Autodesk Inventor part; units mm, degrees
ref_plane "工作平面2" through (11.9199, 26.93, -12.8525) normal (0, 0, 1) x (-1, 0, 0)
ref_plane "工作平面3" through (0.201, 1.0367, -16.3525) normal (0, 0, -1) x (0, 1, 0)
ref_plane "YZ Plane" through (0, 0, 0) normal (1, 0, 0) x (0, 1, 0)
sketch "草图1" plane through (0, 0, 0) normal (0, 0, 1) x (1, 0, 0)
  line L0 (4.75, -1.5) -> (-4.75, -1.5)
  line L1 (-4.75, -1.5) -> (-4.75, 1.5)
  line L2 (-4.75, 1.5) -> (4.75, 1.5)
  line L3 (4.75, 1.5) -> (4.75, -1.5)
  line L4 (4.75, -1.5) -> (-4.75, 1.5) construction
  line L5 (-4.75, -1.5) -> (4.75, 1.5) construction
  circle A0 centre (0, 0) radius 1
  dimension "d0" = 3
  dimension "d1" = 2
  dimension "d2" = 9.5
extrude "拉伸1" add sketch "草图1" along normal blind 3
sketch "草图2" plane through (0, 0, 3) normal (0, 0, 1) x (1, 0, 0)
  line L0 (4.75, 1.5) -> (-4.75, 1.5)
  line L1 (-4.75, 1.5) -> (-4.75, -1.5)
  line L2 (-4.75, -1.5) -> (4.75, -1.5)
  line L3 (4.75, -1.5) -> (4.75, 1.5)
  circle A0 centre (0, 0) radius 1
extrude "拉伸2" add sketch "草图2" along normal blind 10 contours L3 L2 L1 L0 | A0
sketch "草图3" plane through (-4.75, 1.5, 0) normal (0, 1, 0) x (1, 0, 0)
  line L0 (-1.5, 0) -> (11, 0)
  line L1 (11, 0) -> (11, -7)
  line L2 (11, -7) -> (-1.5, -7)
  line L3 (-1.5, -7) -> (-1.5, 0)
  line L4 (9.5, 0) -> (9.5, -13)
  line L5 (0, 0) -> (0, -13)
  line L6 (9.5, 0) -> (0, 0)
  point P0 (4.75, 0)
  point P1 (-1.5, -3.5)
  point P2 (9.5, -7)
  point P3 (0, -7)
  dimension "d8" = 1.5
  dimension "d9" = 1.5
  dimension "d15" = 7
extrude "拉伸3" add sketch "草图3" against normal blind 3
move faces "移动1" translate (0, 0, 2) faces at (1.5833, 0.5, 13)
sketch "草图4" plane through (0, 0, 0) normal (0, 0, -1) x (-1, 0, 0)
  circle A0 centre (0, 0) radius 1.5
  dimension "d16" = 3
extrude "拉伸4" add sketch "草图4" along normal blind 0.5
ref_plane "工作平面1" through (11.9199, 26.93, -22.8525) normal (0, 0, 1) x (-1, 0, 0)
sketch "草图5" plane through (11.9199, 26.93, -22.8525) normal (0, 0, 1) x (-1, 0, 0)
  circle A0 centre (13.6237, 30.1067) radius 1.5
  circle A1 centre (13.716, 24.2534) radius 1.5
  circle A2 centre (13.6237, 30.1067) radius 1.5
  point P0 (11.9199, 26.93)
  dimension "d19" = 3
sketch "草图7" plane through (0, 0, -0.5) normal (0, 0, -1) x (-1, 0, 0)
  circle A0 centre (0, 0) radius 1.5
ref_plane "工作平面2" through (11.9199, 26.93, -12.8525) normal (0, 0, 1) x (-1, 0, 0)
sketch "草图8" plane through (11.9199, 26.93, -12.8525) normal (0, 0, 1) x (-1, 0, 0)
  circle A0 centre (12.3625, 23.27) radius 1.5
  point P0 (11.9199, 26.93)
sketch "草图9" plane through (0, 0, 0) normal (1, 0, 0) x (0, 1, 0)
  line L0 (-4.6767, -22.8525) -> (-1.6767, -22.8525)
  line L1 (-3.1767, -22.8525) -> (-3.1767, -11.5324)
  arc A0 (-1.651, -7.3854) -> (-3.1767, -11.5324) centre (3.2225, -11.5324) ccw
  arc A1 (-1.651, -7.3854) -> (0.0125, -4.1729) centre (-6.1762, -3.0051) ccw
  point P0 (-3.6148, -22.5313)
  point P1 (-2.7659, -4.1729)
sweep "扫掠1" add profiles "草图5" path "草图9" path curves L1 A0 A1 contours A0
loft "放样1" add section 1 edges at (1.5, 0, -0.5) section 2 edges at (-0.2038, 0.0125, -4.1729)
sketch "草图15" plane through (0, 0, 0) normal (0, 0, -1) x (-1, 0, 0)
  line L0 (-6.25, 1.5) -> (0, 1.5)
  line L1 (4.75, -1.5) -> (6.25, -1.5)
  line L2 (-6.25, 1.5) -> (6.25, 1.5)
  line L3 (6.25, 1.5) -> (6.25, -1.5)
  line L4 (6.25, -1.5) -> (-6.25, -1.5)
  line L5 (-6.25, -1.5) -> (-6.25, 1.5)
  point P0 (0, 0)
  point P1 (0, 1.5)
extrude "拉伸9" add sketch "草图15" along normal blind 8
sketch "草图16" plane through (4.75, 1.5, 7) normal (0, 1, 0) x (1, 0, 0)
  line L0 (1.5, 15) -> (-11, 15)
  line L1 (1.5, 15) -> (-4.829, 15)
  line L2 (-4.829, 15) -> (-4.829, 4.4703)
  line L3 (-4.829, 4.4703) -> (1.5, 4.4703)
  line L4 (1.5, 4.4703) -> (1.5, 15)
  point P0 (-4.75, 7)
extrude "拉伸10" cut sketch "草图16" against normal blind 6.75
sketch "草图17" plane through (-1.7038, -3.1767, -22.8525) normal (0, 0, -1) x (-1, 0, 0)
  circle A0 centre (0, 0) radius 1.5
  circle A1 centre (0, 0) radius 1
  point P0 (-1.7038, 3.1767)
  dimension "d46" = 2
ref_plane "工作平面3" through (0.201, 1.0367, -16.3525) normal (0, 0, -1) x (0, 1, 0)
extrude "拉伸11" cut sketch "草图17" against normal up to surface (6.5 mm away)
sketch "草图18" plane through (-1.7038, -3.1767, -16.3525) normal (0, 0, -1) x (-1, 0, 0)
  circle A0 centre (0, 0) radius 1
  point P0 (-1.7038, 3.1767)
extrude "拉伸12" add sketch "草图18" along normal blind 9.5
chamfer "倒角2" distance 0.5 angle 45 1 edges at (-0.7038, -3.1767, -25.8525)
offset faces "大小2" outward -3.5 faces at (1.5833, -0.5, 15)
offset faces "大小3" outward 2 faces at (1.5833, -0.5, 11.5)
properties part number "轴系按钮2"
Here's how the part is built. I have some questions about the finished solid (model axes, mm). A direction names the side the tool comes from. Coordinates: 2 decimals unless noted, no trailing zeros. Write each loop counter-clockwise with the first axis right and the second up, starting at its lowest first coordinate (ties: lowest second). Pieces come first, ordered by that corner, then holes.
1) If we section it at B-B (z = 1.5): List the corners of the cut face in (x, y) for me.
Filled in:
outline: (-6.25, -1.5) - (-0.08, -1.5) - (-0.08, 1.5) - (-6.25, 1.5) - close
2) If we section it at C-C (x = -4.25): List the corners of the cut face in (y, z) for me.
Filled in:
outline: (-1.5, -8) - (1.5, -8) - (1.5, 13.5) - (-1.5, 13.5) - close
3) If we section it at A-A (y = 1): List the corners of the cut face in (x, z) for me.
Filled in:
outline: (-6.25, -8) - (-0.08, -8) - (-0.08, 2.53) - (6.25, 2.53) - (6.25, 7) - (4.75, 7) - (4.75, 13.5) - (-4.75, 13.5) - (-4.75, 7) - (-6.25, 7) - close
4) If we section it at D-D (z = -15): List the corners of the cut face in (x, y) for me, plus the area to 3 significant figures.
Filled in:
outline: circle Ø3 at (-1.7, -3.18)
area: 7.07 mm2
5) Which directions (+Z, -Z, +X, -X, +Y, -Y) give clear straight access to the entire face, cutting with the end or side of a thin tool? Please do faces 1 (the face through (-0.079, 0, -3)), 2 (the face through (-2.17, -2.29, -20.79)), 3 (the face through (-5, 0, 7)).
Filled in:
face 1: -Z, +X, +Y, -Y
face 2: -Z
face 3: +Z, -X, +Y, -Y
6) If I drill on line 1 (Z direction, x = 5.5, y = 1.25); line 2 (Z direction, x = 4.5, y = -0.75); line 3 (X direction, y = -1, z = 1), over which ranges is the centre line in solid material (lowest first)?
Filled in:
line 1: z = 2.53 to 7
line 2: z = 2.53 to 13.5
line 3: x = -6.25 to -0.08
7) I'm going to push flat-ended pins straight in: pin 1 (2.5 mm diameter, centred on y = 0.5, z = 10.5, fed in from +X); pin 2 (2.5 mm diameter, centred on y = -0.5, z = -1, fed in from +X); pin 3 (6.5 mm diameter, centred on x = 0, z = -1.5, fed in from -Y); pin 4 (2 mm diameter, centred on x = 0, z = 0, fed in from +Y). Where does each tip first touch, or does it pass through?
Filled in:
pin 1: stops at x = 4.75
pin 2: stops at x = -0.08
pin 3: stops at y = -1.57
pin 4: stops at y = 1.5
